from build123d import *

# Parameters (mm, degrees)
F0_W     = 167
F0_H     = 95
F0_R     = 2
F0_R_2   = 11.05
F0_W_2   = 75
F0_H_2   = 20
F1_DEPTH = 0.75
F2_R     = 5
F3_R     = 5
F4_SIZE  = 0.5


# Not quite as in the source:
# - a feature names something its author has since deleted; it is built from what else it names


with BuildPart() as f1:
    # F0 (on Top) → F1 (new body, symmetric)
    with BuildSketch(Plane.XY):
        with Locations((36.5, 0)):
            Rectangle(F0_W, F0_H)
        with Locations((-25.5706578493, -29.7)):
            Circle(F0_R, mode=Mode.SUBTRACT)
        with Locations((0, -29.7)):
            Circle(F0_R_2, mode=Mode.SUBTRACT)
        with Locations((24.4293421507, -29.7)):
            Circle(F0_R, mode=Mode.SUBTRACT)
        with Locations((75, -29.7)):
            Rectangle(F0_W_2, F0_H_2, mode=Mode.SUBTRACT)
        Circle(F0_R_2, mode=Mode.SUBTRACT)
        with Locations((-25, 29.7)):
            Circle(F0_R, mode=Mode.SUBTRACT)
        with Locations((0, 29.7)):
            Circle(F0_R_2, mode=Mode.SUBTRACT)
        with Locations((25, 29.7)):
            Circle(F0_R, mode=Mode.SUBTRACT)
        with Locations((75, 0)):
            Rectangle(F0_W_2, F0_H_2, mode=Mode.SUBTRACT)
        with Locations((75, 29.7)):
            Rectangle(F0_W_2, F0_H_2, mode=Mode.SUBTRACT)
    extrude(amount=F1_DEPTH, both=True)

    # F2
    f2_edges = [f1.edges().sort_by_distance(p)[0] for p in [
        (120, 47.5, 0),
        (120, -47.5, 0),
        (-47, -47.5, 0),
        (-47, 47.5, 0),
    ]]
    fillet(f2_edges, radius=F2_R)

    # F3
    f3_edges = [f1.edges().sort_by_distance(p)[0] for p in [
        (37.5, 39.7, 0),
        (37.5, 10, 0),
        (37.5, -19.7, 0),
        (112.5, 39.7, 0),
        (112.5, 10, 0),
        (112.5, -19.7, 0),
        (112.5, -39.7, 0),
        (112.5, -10, 0),
        (112.5, 19.7, 0),
        (37.5, -39.7, 0),
        (37.5, -10, 0),
        (37.5, 19.7, 0),
    ]]
    fillet(f3_edges, radius=F3_R)

    # F4
    f4_edges = [f1.edges().sort_by_distance(p)[0] for p in [
        (-27.570658, -29.7, -0.75),
        (22.429342, -29.7, -0.75),
        (23, 29.7, -0.75),
        (-27, 29.7, -0.75),
    ]]
    chamfer(f4_edges, length=F4_SIZE)


solid = f1.part
Read the model definition and answer for the solid it produces. Units are mm, in the model's axes. Give positions to 0.01 mm unless a question says otherwise; leave off trailing zeros. Write each loop counter-clockwise with the first axis right and the second up, starting at its lowest first coordinate (ties: lowest second). Pieces come first, ordered by that corner, then holes. Notation, with made-up numbers: (36, 66.5) -> (86, 66.5) arc R20 ccw to (86, 92.5) -> close; hole circle Ø10 at (56, 32.25). An arc over 180 degrees is marked (long way). Answer as a JSON object with one key per item and string values. Group by question number.
1) This flat-tipped pin is pushed along its axis until it touches: P1, Ø13.5, axis at x = 0, y = -29.7, coming from the -Z side (3 decimals). Where does it stop, or does it pass through?
2) The mould has two halves that part along X. Classify faces 1 (the cylindrical face through (-45.57, 46, -0.01)), 2 (the flat face through (17, 1, -0.75)), 3 (the cylindrical face through (24.169, -27.717, 0.243)): +X half, -X half, draft (parallel to the pull), parting line (faces both ways), or undercut.
3) Find section A-A (y = -29.7). Write down the section's boundary in (x, z), and give its area (4 significant figures).
4) Find section B-B (x = 48). Write down the section's boundary in (y, z), and give its area (3 significant figures).
5) Find section C-C (y = 0). Write down the section's boundary in (x, z), and give its area (3 significant figures).
6) Find section D-D (z = 0.4). Count the separate pieces of the cut face and the enclosed holes in it, and give its area (3 significant figures).
7) Consider L1, parallel to Y at x = 0, z = -0.05; L2, parallel to X at y = 25, z = 0.5; L3, parallel to Y at x = 68.5, z = 0.2. Determine where each line is inside the solid, lowest interval first. Write a range as from..to.
Values follow:
{
 "1": {"P1": "passes through"},
 "2": {"face 1": "-X half", "face 2": "draft", "face 3": "undercut"},
 "3": {"outline": "(-47, -0.75) -> (-28.07, -0.75) -> (-27.57, -0.25) -> (-27.57, 0.75) -> (-47, 0.75) -> close; (-23.57, -0.25) -> (-23.07, -0.75) -> (-11.05, -0.75) -> (-11.05, 0.75) -> (-23.57, 0.75) -> close; (11.05, -0.75) -> (21.93, -0.75) -> (22.43, -0.25) -> (22.43, 0.75) -> (11.05, 0.75) -> close; (26.43, -0.25) -> (26.93, -0.75) -> (37.5, -0.75) -> (37.5, 0.75) -> (26.43, 0.75) -> close; (112.5, -0.75) -> (120, -0.75) -> (120, 0.75) -> (112.5, 0.75) -> close", "area": "92.35 mm2"},
 "4": {"outline": "(-47.5, -0.75) -> (-39.7, -0.75) -> (-39.7, 0.75) -> (-47.5, 0.75) -> close; (-19.7, -0.75) -> (-10, -0.75) -> (-10, 0.75) -> (-19.7, 0.75) -> close; (10, -0.75) -> (19.7, -0.75) -> (19.7, 0.75) -> (10, 0.75) -> close; (39.7, -0.75) -> (47.5, -0.75) -> (47.5, 0.75) -> (39.7, 0.75) -> close", "area": "52.5 mm2"},
 "5": {"outline": "(-47, -0.75) -> (-11.05, -0.75) -> (-11.05, 0.75) -> (-47, 0.75) -> close; (11.05, -0.75) -> (37.5, -0.75) -> (37.5, 0.75) -> (11.05, 0.75) -> close; (112.5, -0.75) -> (120, -0.75) -> (120, 0.75) -> (112.5, 0.75) -> close", "area": "105 mm2"},
 "6": {"separate pieces": "1", "enclosed holes": "10", "area": "10,200 mm2"},
 "7": {"L1": "y = -47.5..-40.75, -18.65..-11.05, 11.05..18.65, 40.75..47.5", "L2": "x = -47..-10, 10..37.5, 112.5..120", "L3": "y = -47.5..-39.7, -19.7..-10, 10..19.7, 39.7..47.5"}
}
